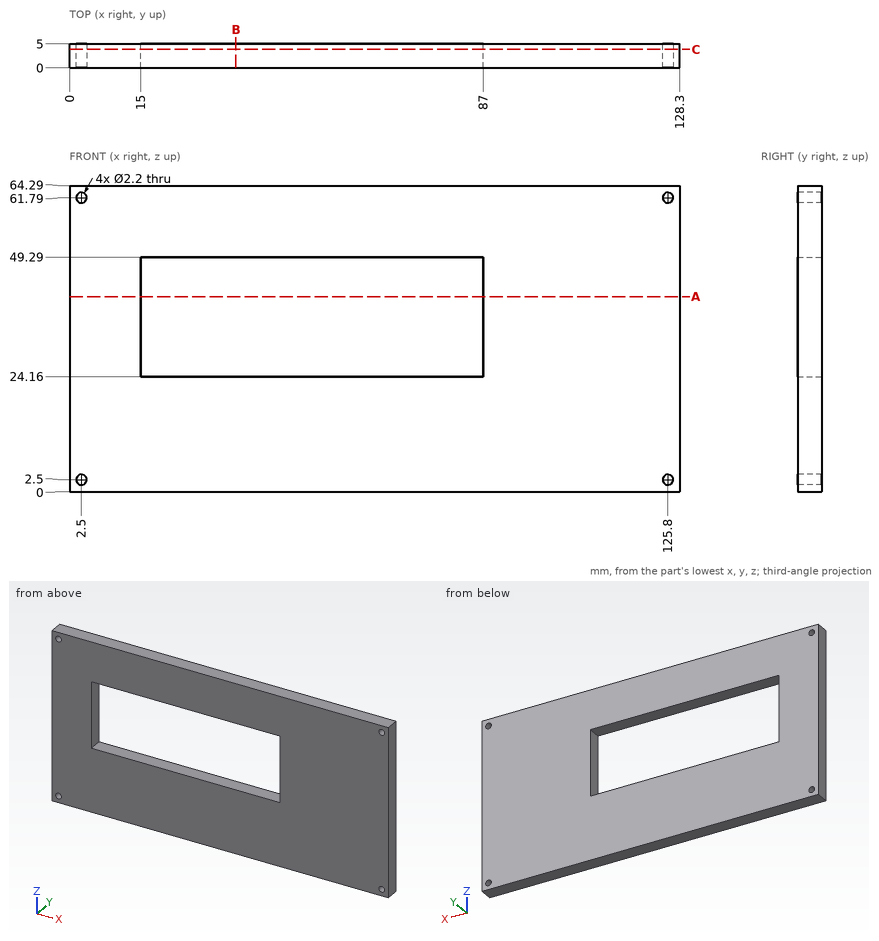
Answer from the drawing. Dimensions are ordinates in mm from the lowest x, y and z of the part. Give positions to 0.01 mm unless a question says otherwise; leave off trailing zeros. Order: outer loops, then holes, each group sorted by start corner. A loop starts at its lowest first (then second) coordinate and runs counter-clockwise, first axis right, second up. Notation, with made-up numbers: (56.5, 76) - (110.5, 76) arc R19 ccw to (110.5, 87) - close; hole circle Ø11 at (71, 19.25). An arc over 180 degrees is marked (long way). One line per item, written item: value. Start each with the question number.
1) A cutting plane is placed at C-C on y = 3.85. Give the vertices of the cut face in (x, z), then the cut area to 3 significant figures.
2) A cutting plane is placed at B-B on x = 35. Give the vertices of the cut face in (y, z).
3) Find the intervals of material crossed by L1, parallel to Z at x = 125.8, y = 2.35; L2, parallel to Z at x = 66, y = 2.3; L3, parallel to X at y = 2.3, z = 25.5, in increasing order.
4) A cutting plane is placed at A-A on z = 41. Give the vertices of the cut face in (x, y), then the cut area to 4 significant figures.
Answer sheet:
1. outline: (0, 0) - (128.3, 0) - (128.3, 64.29) - (0, 64.29) - close; hole circle Ø2.2 at (2.5, 2.5); hole circle Ø2.2 at (2.5, 61.79); hole (15, 24.16) - (87, 24.16) - (87, 49.29) - (15, 49.29) - close; hole circle Ø2.2 at (125.8, 2.5); hole circle Ø2.2 at (125.8, 61.79)
1. area: 6,420 mm2
2. outline: (0, 0) - (5, 0) - (5, 24.16) - (0, 24.16) - close; (0, 49.29) - (5, 49.29) - (5, 64.29) - (0, 64.29) - close
3. L1: z = 0 to 1.4, 3.6 to 60.69, 62.89 to 64.29
3. L2: z = 0 to 24.16, 49.29 to 64.29
3. L3: x = 0 to 15, 87 to 128.3
4. outline: (0, 0) - (15, 0) - (15, 5) - (0, 5) - close; (87, 0) - (128.3, 0) - (128.3, 5) - (87, 5) - close
4. area: 281.5 mm2
